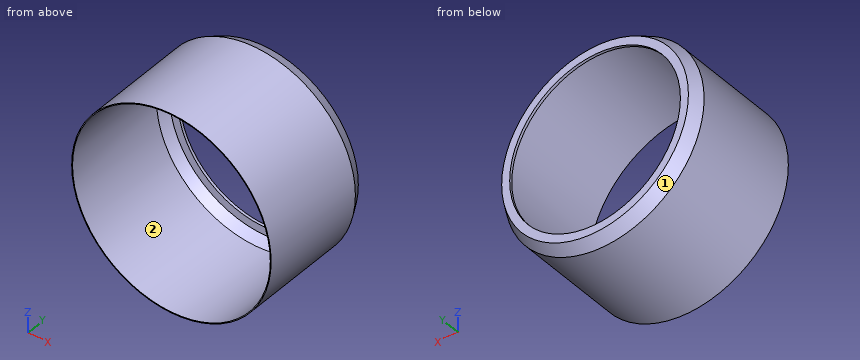
```python
from build123d import *

# Parameters (mm, degrees)
SKETCH_1_R      = 35
SKETCH_1_R_2    = 32
EXTRUDE_1_DEPTH = 1


with BuildPart() as part:
    # 草图1 → 凸台-拉伸1 (new body)
    with BuildSketch(Plane(origin=(0, 0, 0), x_dir=(1, 0, 0), z_dir=(0, 1, 0))):
        Circle(SKETCH_1_R)
        Circle(SKETCH_1_R_2, mode=Mode.SUBTRACT)
    extrude(amount=EXTRUDE_1_DEPTH)

    # 草图2 → 旋转1 (revolve)
    with BuildSketch(Plane.XY):
        Polygon((35, 1), (37.395208955, -3.470302207), (37.395208955, -43.771735553), (37.072710077, -43.771735553), (37.072710077, -3.643098623), (35, 0.549668864), align=None)
    revolve(axis=Axis((0, 0, 0), (0, -1, 0)))


solid = part.part
```
The listing builds one solid part. Answer for the finished solid, in the listing's coordinates (mm). Face numbers are marked on the shaded views. Round coordinates to 2 decimals unless told otherwise and drop trailing zeros. Loops run counter-clockwise (first coordinate to the right, second up) from the corner with the lowest first, then second, coordinate; pieces in that order, holes last.
Q1. Find the intervals of material crossed by line 1 (Z direction, x = 0, y = -23); line 2 (X direction, y = -2.5, z = 5); line 3 (Z direction, x = 0, y = 0.2), in increasing order.
Q2. For a pull along X with two mould halves and no side action, classify the marked faces 1 and 2 as released by +X, released by -X, zero draft, split by the parting line, or undercut.
Q3. Section A-A, the plane x = 0 is taken. Determine the outline of the cut face in (y, z).
Q4. Section B-B, the plane z = 0 is taken. Determine the outline of the cut face in (x, y), then the cut area to 3 significant figures.
Q5. Given pin 1 Ø1.5 at (y, z) = (-29.5, -4) entering from -X; pin 2 Ø1 at (x, y) = (15, -9.5) entering from +Z; pin 3 Ø6 at (y, z) = (-10.5, -29.5) entering from +X, each flat-ended and moving along its own axis, determine where each tip first touches the part or whether it passes through.
Q6. Section C-C, the plane y = -35 is taken. Determine the outline of the cut face in (x, z).
Completed:
1. line 1: z = -37.4 to -37.07, 37.07 to 37.4
1. line 2: x = -36.53 to -36.16, 36.16 to 36.53
1. line 3: z = -35.43 to -35.17, -35 to -32, 32 to 35, 35.17 to 35.43
2. face 1: split by the parting line
2. face 2: undercut
3. outline: (-43.77, -37.4) - (-3.47, -37.4) - (1, -35) - (1, -32) - (0, -32) - (0, -35) - (0.55, -35) - (-3.64, -37.07) - (-43.77, -37.07) - close; (-43.77, 37.07) - (-3.64, 37.07) - (0.55, 35) - (0, 35) - (0, 32) - (1, 32) - (1, 35) - (-3.47, 37.4) - (-43.77, 37.4) - close
4. outline: (-37.4, -43.77) - (-37.07, -43.77) - (-37.07, -3.64) - (-35, 0.55) - (-35, 0) - (-32, 0) - (-32, 1) - (-35, 1) - (-37.4, -3.47) - close; (32, 0) - (35, 0) - (35, 0.55) - (37.07, -3.64) - (37.07, -43.77) - (37.4, -43.77) - (37.4, -3.47) - (35, 1) - (32, 1) - close
4. area: 34.7 mm2
5. pin 1: stops at x = -37.25
5. pin 2: stops at z = 34.47
5. pin 3: stops at x = 26.38
6. outline: circle Ø74.79 at (0, 0); hole circle Ø74.15 at (0, 0)
